Here's how the part is built. I have some questions about the finished solid (model axes, mm). Face numbers are marked on the shaded views. A direction names the side the tool comes from. Give positions to 0.01 mm unless a question says otherwise; leave off trailing zeros. Loops run counter-clockwise (first coordinate to the right, second up) from the corner with the lowest first, then second, coordinate; pieces in that order, holes last.
Q1. If we section it at C-C (y = 9.5): Please give me the cut outline in (x, z).
Q2. If we section it at A-A (z = 3.7): Please give me the cut outline in (x, y), plus the area to 3 significant figures.
Q3. We'd pull the mould along X, two halves only. Please class the marked faces 3, 4 and 5: +X half, -X half, draft (parallel to the pull), parting line (faces both ways), or undercut.
Q4. If we section it at B-B (x = 0.25): Please give me the cut outline in (y, z).
Q5. I need wall thicknesses on line 1 (Z direction, x = -7, y = -3.95); line 2 (Y direction, x = 1, z = 0.7); line 3 (Y direction, x = -0.25, z = 3.65). Which ranges of each line are inside material? Lowest first, please.
Q6. Will these pins go through, and if not, where does the flat tip stop? P1, Ø1.2, axis at x = 7, z = 2, coming from the -Y side; P2, Ø2, axis at y = 13, z = 3.5, coming from the -X side; P3, Ø1.2, axis at x = -7, z = 2, coming from the +Y side.
Q7. If we section it at D-D (z = 2.25): Please give me the cut outline in (x, y).
Q8. For the marked faces 1 and 2, which set-ups out of +Z, -Z, +X, -X, +Y, -Y let a thin tool reach every point of the face, with its end or its side?
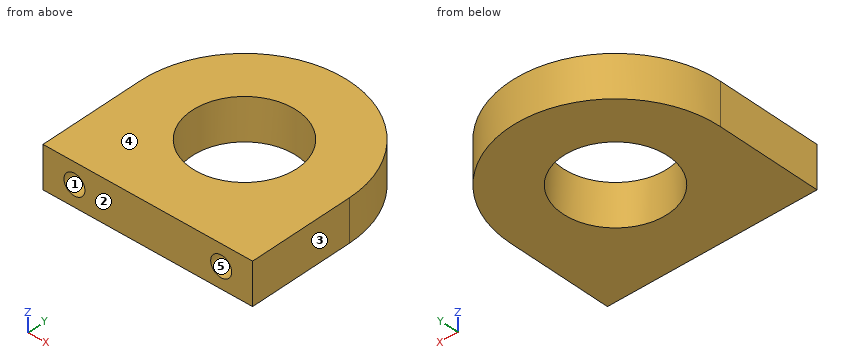
from build123d import *

# Parameters (mm, degrees)
SKETCH1_R           = 5
BOSS_EXTRUDE1_DEPTH = 4
SKETCH2_R           = 1
CUT_EXTRUDE1_DEPTH  = 4


with BuildPart() as part:
    # Sketch1 → Boss-Extrude1 (new body)
    with BuildSketch(Plane.XY):
        with BuildLine():
            Line((-10, -5), (10, -5))
            Line((10, -5), (10, 5))
            ThreePointArc((10, 5), (0, 15), (-10, 5))
            Line((-10, 5), (-10, -5))
        make_face()
        with Locations((0, 5)):
            Circle(SKETCH1_R, mode=Mode.SUBTRACT)
    extrude(amount=BOSS_EXTRUDE1_DEPTH)

    # Sketch2 → Cut-Extrude1 (cut)
    with BuildSketch(Plane.XZ.offset(5)):
        with Locations((-7, 2)):
            Circle(SKETCH2_R)
        with Locations((7, 2)):
            Circle(SKETCH2_R)
    extrude(amount=-CUT_EXTRUDE1_DEPTH, mode=Mode.SUBTRACT)


solid = part.part
Check sheet entries:
1. outline: (-8.93, 0) - (-2.18, 0) - (-2.18, 4) - (-8.93, 4) - close; (2.18, 0) - (8.93, 0) - (8.93, 4) - (2.18, 4) - close
2. outline: (-10, -5) - (10, -5) - (10, 5) arc R10 ccw to (-10, 5) - close; hole circle Ø10 at (0, 5)
2. area: 279 mm2
3. face 3: +X half
3. face 4: draft
3. face 5: undercut
4. outline: (-5, 0) - (0.01, 0) - (0.01, 4) - (-5, 4) - close; (9.99, 0) - (15, 0) - (15, 4) - (9.99, 4) - close
5. line 1: z = 0 to 1, 3 to 4
5. line 2: y = -5 to 0.1, 9.9 to 14.95
5. line 3: y = -5 to 0.01, 9.99 to 15
6. P1: stops at y = -1
6. P2: stops at x = -7.14
6. P3: stops at y = 12.68
7. outline: (-10, -5) - (-7.97, -5) - (-7.97, -1) - (-6.03, -1) - (-6.03, -5) - (6.03, -5) - (6.03, -1) - (7.97, -1) - (7.97, -5) - (10, -5) - (10, 5) arc R10 ccw to (-10, 5) - close; hole circle Ø10 at (0, 5)
8. face 1: -Y
8. face 2: +Z, -Z, +X, -X, -Y
